Verification items for the finished model (mm, model axes). A direction names the side the tool comes from. Give positions to 0.01 mm unless a question says otherwise; leave off trailing zeros. Loops run counter-clockwise (first coordinate to the right, second up) from the corner with the lowest first, then second, coordinate; pieces in that order, holes last. Notation, with made-up numbers: (49, 37.25) - (88, 37.25) arc R16 ccw to (88, 44.25) - close; hole circle Ø6 at (63, 67). An arc over 180 degrees is marked (long way). One line per item, written item: value. Start each with the question number.
1. Sectioned sample at B-B (y = 18.5). Record the cut outline in (x, z).
2. Scan lines: L1, parallel to X at y = 23, z = 7.75; L2, parallel to Y at x = -27.5, z = 2.75; L3, parallel to X at y = 18, z = 3.25. Record each from-to range of solid material in increasing order. Write a range as [from, to].
3. Gauge pin test, flat ends, axial feed: pin 1 (5 mm diameter, centred on y = 14, z = 6, fed in from -X); pin 2 (6 mm diameter, centred on x = -18, z = 8.5, fed in from +Y); pin 3 (1.5 mm diameter, centred on x = -32, z = 1.5, fed in from +Y). Record the tip position at first contact, or that the pin passes through.
4. Sectioned sample at D-D (x = -31.5). Record the cut outline in (y, z), plus the area to 3 significant figures.
5. Sectioned sample at C-C (z = 6.75). Record the cut outline in (x, y).
6. Mould release check, pull along X, two halves, no side actions. Record for faces 6 (the cylindrical face through (-16.353, 19.981, 4.93)), 7 (the flat face through (-7.721, 19.534, 4.93)), 8 (the flat face through (-26.8, 38.64, 4.93)), 9 (the flat face through (-24, 31, 10)): pulls with the +X half, pulls with the -X half, needs draft (parallel to the pull), parting line crosses it, or undercut.
7. Sectioned sample at A-A (x = -26.5). Record the cut outline in (y, z), plus the area to 3 significant figures.
8. Access from +Z, -Z, +X, -X, +Y, -Y to the whole of each face (thin tool, end or side, straight path). Record for faces 1 (the flat face through (-9.781, 14, 5)), 2 (the flat face through (-23, 5.389, 5)), 3 (the flat face through (-9.781, 32, 5)), 4 (the flat face through (-36.781, 15, 5)), 5 (the flat face through (-5.603, 23, 5)).
from build123d import *

# Parameters (mm, degrees)
F0_R     = 7.5
F1_DEPTH = 10
F2_SIZE  = 2
F3_SIZE  = 2


with BuildPart() as f1:
    # F0 (on Top) → F1 (new body)
    with BuildSketch(Plane.XY):
        Polygon((-23.2808627188, 42.1585307921), (-28.9580689277, 36.4813245833), (-17.60365651, 36.4813245833), align=None)
        Polygon((-4.1889796268, 23.0666477001), (-9.7808627188, 28.6585307921), (-9.7808627188, 17.4747646081), align=None)
        Polygon((-17.7743027436, 9.4813245833), (-28.787422694, 9.4813245833), (-23.2808627188, 3.9747646081), align=None)
        Polygon((-17.60365651, 36.4813245833), (-28.9580689277, 36.4813245833), (-36.7808627188, 28.6585307921), (-36.7808627188, 17.4747646081), (-28.787422694, 9.4813245833), (-17.7743027436, 9.4813245833), (-9.7808627188, 17.4747646081), (-9.7808627188, 28.6585307921), align=None)
        with Locations((-23.2808627188, 22.8532869369)):
            Circle(F0_R, mode=Mode.SUBTRACT)
        Polygon((-36.7808627188, 17.4747646081), (-36.7808627188, 28.6585307921), (-42.3727458109, 23.0666477001), align=None)
        Polygon((-9.7808627188, 36.4813245833), (-17.60365651, 36.4813245833), (-9.7808627188, 28.6585307921), align=None)
        Polygon((-28.9580689277, 36.4813245833), (-36.7808627188, 36.4813245833), (-36.7808627188, 28.6585307921), align=None)
        Polygon((-28.787422694, 9.4813245833), (-36.7808627188, 17.4747646081), (-36.7808627188, 9.4813245833), align=None)
        Polygon((-9.7808627188, 9.4813245833), (-9.7808627188, 17.4747646081), (-17.7743027436, 9.4813245833), align=None)
    extrude(amount=F1_DEPTH)

    # F2
    f2_edges = [f1.edges().sort_by_distance(p)[0] for p in [
        (-4.18898, 23.066648, 5),
    ]]
    chamfer(f2_edges, length=F2_SIZE)

    # F3
    f3_edges = [f1.edges().sort_by_distance(p)[0] for p in [
        (-9.780863, 9.481325, 5),
        (-23.280863, 3.974765, 5),
        (-36.780863, 9.481325, 5),
        (-9.780863, 36.481325, 5),
        (-23.280863, 42.158531, 5),
        (-36.780863, 36.481325, 5),
        (-42.372746, 23.066648, 5),
    ]]
    chamfer(f3_edges, length=F3_SIZE)


solid = f1.part
Results are:
1. outline: (-37.81, 0) - (-29.39, 0) - (-29.39, 10) - (-37.81, 10) - close; (-17.17, 0) - (-8.76, 0) - (-8.76, 10) - (-17.17, 10) - close
2. L1: x = [-40.96, -30.78], [-15.78, -5.6]
2. L2: y = [8.19, 16.65], [29.05, 37.94]
2. L3: x = [-37.31, -29], [-17.56, -9.26]
3. pin 1: stops at x = -36.78
3. pin 2: stops at y = 39.88
3. pin 3: stops at y = 36.48
4. outline: (9.48, 0) - (36.48, 0) - (36.48, 10) - (9.48, 10) - close
4. area: 270 mm^2
5. outline: (-40.96, 21.65) - (-36.78, 17.47) - (-36.78, 11.48) - (-34.78, 9.48) - (-28.79, 9.48) - (-24.7, 5.39) - (-21.87, 5.39) - (-17.77, 9.48) - (-11.78, 9.48) - (-9.78, 11.48) - (-9.78, 17.47) - (-5.6, 21.65) - (-5.6, 24.48) - (-9.78, 28.66) - (-9.78, 34.48) - (-11.78, 36.48) - (-17.6, 36.48) - (-21.87, 40.74) - (-24.7, 40.74) - (-28.96, 36.48) - (-34.78, 36.48) - (-36.78, 34.48) - (-36.78, 28.66) - (-40.96, 24.48) - close; hole circle Ø15 at (-23.28, 22.85)
6. face 6: undercut
6. face 7: pulls with the +X half
6. face 8: pulls with the -X half
6. face 9: needs draft
7. outline: (7.19, 0) - (16.08, 0) - (16.08, 10) - (7.19, 10) - close; (29.63, 0) - (38.94, 0) - (38.94, 10) - (29.63, 10) - close
7. area: 182 mm^2
8. face 1: +Z, -Z, +X, -Y
8. face 2: +Z, -Z, +X, -X, -Y
8. face 3: +Z, -Z, +X, +Y
8. face 4: +Z, -Z, -X, -Y
8. face 5: +Z, -Z, +X, +Y, -Y
